from build123d import *

# Parameters (mm, degrees)
SKETCH1_W                = 58
SKETCH1_H                = 52.25
SKETCH1_R                = 0.65
BOSS_EXTRUDE1_DEPTH      = 0.8
SKETCH1_3_W              = 5.7
SKETCH1_3_H              = 19.65
SKETCH1_3_W_2            = 8.5
SKETCH1_3_H_2            = 5.1
BOSS_EXTRUDE2_DEPTH      = 7.92
SKETCH1_4_W              = 18.1
SKETCH1_4_H              = 20.1
SKETCH1_4_H_2            = 5.5
BOSS_EXTRUDE3_DEPTH      = 2
BOSS_EXTRUDE4_DEPTH      = 8.2
BOSS_EXTRUDE4_DEPTH_BACK = 5.7
BOSS_EXTRUDE4_START      = -0.8
SKETCH1_5_W              = 5.047957292
SKETCH1_5_H              = 5.27600609


with BuildPart() as part:
    # Sketch1 → Boss-Extrude1 (new body)
    with BuildSketch(Plane(origin=(0, 0, 0), x_dir=(1, 0, 0), z_dir=(0, 1, 0))):
        with Locations((29, 26.125)):
            Rectangle(SKETCH1_W, SKETCH1_H)
        with Locations(Location((2.1, 1.85, 0), (0, 0, 270))):
            Circle(SKETCH1_R, mode=Mode.SUBTRACT)
        with Locations(Location((56.05, 1.75, 0), (0, 0, 270))):
            Circle(SKETCH1_R, mode=Mode.SUBTRACT)
        with Locations(Location((55.7, 50.3, 0), (0, 0, 270))):
            Circle(SKETCH1_R, mode=Mode.SUBTRACT)
    extrude(amount=-BOSS_EXTRUDE1_DEPTH)

    # Sketch1<3> → Boss-Extrude2 (add)
    with BuildSketch(Plane(origin=(0, 0, 0), x_dir=(1, 0, 0), z_dir=(0, 1, 0))):
        with Locations((2.85, 28.425)):
            Rectangle(SKETCH1_3_W, SKETCH1_3_H)
        Polygon((-4.3, 18.6), (0, 18.6), (0, 38.25), (-4.3, 38.25), (-4.3, 35.25), (-4.3, 30.15), align=None)
        with Locations((-8.55, 32.7)):
            Rectangle(SKETCH1_3_W_2, SKETCH1_3_H_2)
    extrude(amount=BOSS_EXTRUDE2_DEPTH)

    # Sketch1<4> → Boss-Extrude3 (add)
    with BuildSketch(Plane(origin=(0, 0, 0), x_dir=(1, 0, 0), z_dir=(0, 1, 0))):
        with Locations((36.15, 10.05)):
            Rectangle(SKETCH1_4_W, SKETCH1_4_H)
        with Locations((36.15, -2.75)):
            Rectangle(SKETCH1_4_W, SKETCH1_4_H_2)
    extrude(amount=BOSS_EXTRUDE3_DEPTH)

    # Sketch1<5> → Boss-Extrude4 (add, two sides: drawn at the far end of the back side and taken through both)
    with BuildSketch(Plane(origin=(0, 0, 0), x_dir=(1, 0, 0), z_dir=(0, 1, 0)).offset(BOSS_EXTRUDE4_START - BOSS_EXTRUDE4_DEPTH_BACK)):
        with Locations((14.523978646, 7.638003045)):
            Rectangle(SKETCH1_5_W, SKETCH1_5_H)
    extrude(amount=BOSS_EXTRUDE4_DEPTH + BOSS_EXTRUDE4_DEPTH_BACK)


solid = part.part
Geometry: final body of the model. Coordinates: model frame, mm. A direction names the side the tool comes from. Round coordinates to 2 decimals unless told otherwise and drop trailing zeros. Loops run counter-clockwise (first coordinate to the right, second up) from the corner with the lowest first, then second, coordinate; pieces in that order, holes last.
Q1. Section D-D on x = 21. Return loops of the section in (y, z).
Q2. Section A-A on y = 4. Return loops of the section in (x, z).
Q3. Pin query (flat end, axial travel): P1, Ø0.9, axis at x = 26, y = -0.5, coming from the +Z side; P2, Ø3, axis at x = 47, z = -29.5, coming from the +Y side; P3, Ø4, axis at y = 2.5, z = -30.5, coming from the +X side. Return the tip coordinate at first contact, or that it passes through.
Q4. Section C-C on z = -26. Return loops of the section in (x, y), plus the area to 3 significant figures.
Q5. Pull-direction query (X, two-part tool) for faces 4 (the flat face through (29, -0.8, -26)), 5 (the flat face through (-4.3, 4, -24)), 6 (the flat face through (45.2, 1, -7)), 7 (the flat face through (17.048, 4, -8)); classes: released by +X, released by -X, zero draft, split by the parting line, or undercut.
Q6. Section B-B on z = -12. Return loops of the section in (x, y), plus the area to 3 significant figures.
Q7. Material intervals for L1, parallel to X at y = -0.6, z = -1.75; L2, parallel to X at y = -0.35, z = -50.3; L3, parallel to Z at x = 56.05, y = -0.55, sorted ascending.
Q8. Access query for faces 1 (the flat face through (36, 0, 3)), 2 (the flat face through (14, -4, -10.276)), 3 (the flat face through (12, 4, -8)). Directions: +Z, -Z, +X, -X, +Y, -Y. A direction counts if a zero-diameter tool reaches every point of the face in a straight line with its end or side. Return the directions, or none.
Evaluation:
1. outline: (-0.8, -52.25) - (0, -52.25) - (0, 0) - (-0.8, 0) - close
2. outline: (-12.8, -35.25) - (-4.3, -35.25) - (-4.3, -38.25) - (5.7, -38.25) - (5.7, -18.6) - (-4.3, -18.6) - (-4.3, -30.15) - (-12.8, -30.15) - close; (12, -10.28) - (17.05, -10.28) - (17.05, -5) - (12, -5) - close
3. P1: stops at z = 0
3. P2: stops at y = 0
3. P3: stops at x = 5.7
4. outline: (-4.3, 0) - (0, 0) - (0, -0.8) - (58, -0.8) - (58, 0) - (5.7, 0) - (5.7, 7.92) - (-4.3, 7.92) - close
4. area: 126 mm2
5. face 4: zero draft
5. face 5: released by -X
5. face 6: released by +X
5. face 7: undercut
6. outline: (0, -0.8) - (58, -0.8) - (58, 0) - (45.2, 0) - (45.2, 2) - (27.1, 2) - (27.1, 0) - (0, 0) - close
6. area: 82.6 mm2
7. L1: x = 0 to 1.46, 2.74 to 55.4, 56.7 to 58
7. L2: x = 0 to 55.05, 56.35 to 58
7. L3: z = -52.25 to -50.85, -49.75 to -2.4, -1.1 to 0
8. face 1: +Z, +X, -X, -Y
8. face 2: -Z, +X, -X, -Y
8. face 3: +Z, -Z, -X, +Y
